Geometry check sheet. Reference: the model listing, model coordinates, mm. A direction names the side the tool comes from. Coordinates: 2 decimals unless noted, no trailing zeros. Write each loop counter-clockwise with the first axis right and the second up, starting at its lowest first coordinate (ties: lowest second). Pieces come first, ordered by that corner, then holes. Notation, with made-up numbers: (83, 48) -> (109, 48) arc R18 cw to (109, 77) -> close; hole circle Ø10 at (39.5, 64). An arc over 180 degrees is marked (long way). Use a Markdown table: item, result.
```python
from build123d import *

# Parameters (mm, degrees)
SKETCH1_R           = 2.25
BOSS_EXTRUDE1_DEPTH = 6
SKETCH2_W           = 3
SKETCH2_H           = 3
CUT_EXTRUDE1_DEPTH  = 7.791538854


with BuildPart() as part:
    # Sketch1 → Boss-Extrude1 (new body)
    with BuildSketch(Plane(origin=(0, 0, 0), x_dir=(1, 0, 0), z_dir=(0, 1, 0))):
        with Locations(Location((0, 0, 0), (0, 0, 270))):
            Circle(SKETCH1_R)
    extrude(amount=BOSS_EXTRUDE1_DEPTH)

    # Sketch2 → Cut-Extrude1 (cut, through all)
    with BuildSketch(Plane(origin=(0, 6, 0), x_dir=(1, 0, 0), z_dir=(0, 1, 0))):
        Rectangle(SKETCH2_W, SKETCH2_H)
    extrude(amount=-CUT_EXTRUDE1_DEPTH, mode=Mode.SUBTRACT)


solid = part.part
```
Item 1: Section check C-C on y = 3.35. Record the boundary of the cut face in (x, z), then the cut area to 3 significant figures.
Answer block:
| item | result |
|---|---|
| outline | circle Ø4.5 at (0, 0); hole (-1.5, -1.5) -> (1.5, -1.5) -> (1.5, 1.5) -> (-1.5, 1.5) -> close |
| area | 6.90 mm^2 |
Item 2: Section check B-B on z = 0. Record the boundary of the cut face in (x, y), then the cut area to 3 significant figures.
Answer block:
| item | result |
|---|---|
| outline | (-2.25, 0) -> (-1.5, 0) -> (-1.5, 6) -> (-2.25, 6) -> close; (1.5, 0) -> (2.25, 0) -> (2.25, 6) -> (1.5, 6) -> close |
| area | 9.00 mm^2 |
Item 3: Section check A-A on x = 0. Record the boundary of the cut face in (y, z), then the cut area to 3 significant figures.
Answer block:
| item | result |
|---|---|
| outline | (0, -2.25) -> (6, -2.25) -> (6, -1.5) -> (0, -1.5) -> close; (0, 1.5) -> (6, 1.5) -> (6, 2.25) -> (0, 2.25) -> close |
| area | 9.00 mm^2 |
Item 4: Tool access check on faces 5 (the flat face through (1.5, 3, 0)), 6 (the flat face through (0, 0, -2)). Record the directions out of +Z, -Z, +X, -X, +Y, -Y that give a thin tool (end or side, any length) a straight path to the whole face; none if there is none.
Answer block:
| item | result |
|---|---|
| face 5 | +Y, -Y |
| face 6 | +Z, -Z, +X, -X, -Y |
Item 5: Section check D-D on z = -1.7. Record the boundary of the cut face in (x, y), then the cut area to 3 significant figures.
Answer block:
| item | result |
|---|---|
| outline | (-1.47, 0) -> (1.47, 0) -> (1.47, 6) -> (-1.47, 6) -> close |
| area | 17.7 mm^2 |
Item 6: Thickness scan on L1, parallel to X at y = 3.15, z = -1.3; L2, parallel to Z at x = -0.65, y = 1.95; L3, parallel to Z at x = -1.05, y = 1.6. Record the ranges inside material, lowest first. Write a range as [from, to].
Answer block:
| item | result |
|---|---|
| L1 | x = [-1.84, -1.5], [1.5, 1.84] |
| L2 | z = [-2.15, -1.5], [1.5, 2.15] |
| L3 | z = [-1.99, -1.5], [1.5, 1.99] |
Item 7: Mould release check, pull along X, two halves, no side actions. Record for faces 1 (the flat face through (0, 6, -2)), 2 (the flat face through (0, 3, 1.5)), 3 (the flat face through (0, 3, -1.5)), 4 (the cylindrical face through (0.676, 2.958, 2.146)): +X half, -X half, draft (parallel to the pull), parting line (faces both ways), or undercut.
Answer block:
| item | result |
|---|---|
| face 1 | draft |
| face 2 | undercut |
| face 3 | undercut |
| face 4 | parting line |
